```python
from build123d import *

# Parameters (mm, degrees)
SKETCH_1_R             = 1.5
EXTRUDE_1_DEPTH        = 8
SKETCH_2_R             = 1
CUT_EXTRUDE_1_DEPTH    = 33
FILLET_1_R             = 2
HOLE_WIZARD_M3_1_D     = 2.5
EXTRUDE_START          = 2.3
SKETCH_8_R             = 4.5
SKETCH_8_R_2           = 1.5
EXTRUDE_2_DEPTH        = 2.3
HOLE_WIZARD_M5_1_D     = 4.2
HOLE_WIZARD_M5_1_DEPTH = 20
HOLE_WIZARD_M5_1_TIP   = 1.2618073
CUT_EXTRUDE_2_DEPTH    = 20


with BuildPart() as part:
    # 草图1 → 凸台-拉伸1 (new body)
    with BuildSketch(Plane.XY):
        with BuildLine():
            Line((0.5, -13), (15.5, -13))
            Line((15.5, -13), (15.5, 13))
            Line((15.5, 13), (0.5, 13))
            Line((0.5, 13), (-4.159282148, 1.717664698))
            ThreePointArc((-4.159282148, 1.717664698), (-4.5, 0), (-4.159282148, -1.717664698))
            Line((-4.159282148, -1.717664698), (0.5, -13))
        make_face()
        Circle(SKETCH_1_R, mode=Mode.SUBTRACT)
    extrude(amount=EXTRUDE_1_DEPTH)

    # 草图2 → 切除-拉伸1 (cut)
    with BuildSketch(Plane.XY.offset(8)):
        with Locations((8.5, 10)):
            Circle(SKETCH_2_R)
        with Locations((8.5, -10)):
            Circle(SKETCH_2_R)
    extrude(amount=-CUT_EXTRUDE_1_DEPTH, mode=Mode.SUBTRACT)

    # 圆角1
    fillet_1_edges = [part.edges().sort_by_distance(p)[0] for p in [
        (0.5, 13, 4),
        (15.5, 13, 4),
        (15.5, -13, 4),
        (0.5, -13, 4),
    ]]
    fillet(fillet_1_edges, radius=FILLET_1_R)

    # M3 螺纹孔1 (through all)
    with Locations(Plane.XY.offset(8)):
        with Locations((8.5, 10), (8.5, -10)):
            Hole(HOLE_WIZARD_M3_1_D / 2)

    # 草图8 → 凸台-拉伸2 (add)
    with BuildSketch(Plane(origin=(0, 0, 0), x_dir=(-1, 0, 0), z_dir=(0, 0, -1)).offset(EXTRUDE_START)):
        Circle(SKETCH_8_R)
        Circle(SKETCH_8_R_2, mode=Mode.SUBTRACT)
    extrude(amount=-EXTRUDE_2_DEPTH)

    # M5 螺纹孔1
    with Locations(Plane.XY.offset(8)):
        with Locations((0, 0)):
            Hole(HOLE_WIZARD_M5_1_D / 2, depth=HOLE_WIZARD_M5_1_DEPTH)
            with Locations((0, 0, -(HOLE_WIZARD_M5_1_DEPTH + HOLE_WIZARD_M5_1_TIP / 2))):  # 118° drill point
                Cone(0, HOLE_WIZARD_M5_1_D / 2, HOLE_WIZARD_M5_1_TIP, mode=Mode.SUBTRACT)

    # 草图12 → 切除-拉伸2 (cut)
    with BuildSketch(Plane(origin=(0, 0, 0), x_dir=(-1, 0, 0), z_dir=(0, 0, -1))):
        with BuildLine():
            Line((-6, 4), (-6, -4))
            ThreePointArc((-6, -4), (-8.5, -6.5), (-11, -4))
            Line((-11, -4), (-11, 4))
            ThreePointArc((-11, 4), (-8.5, 6.5), (-6, 4))
        make_face()
    extrude(amount=-CUT_EXTRUDE_2_DEPTH, mode=Mode.SUBTRACT)


solid = part.part
```
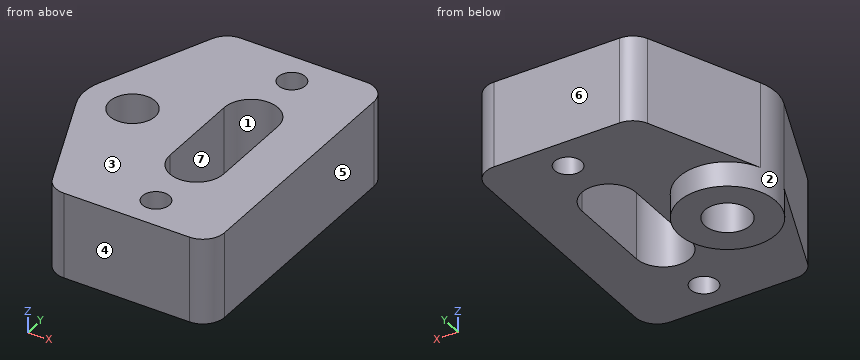
Input: part model. Units: mm. Frame: model coordinates. Face numbers are marked on the shaded views. A direction names the side the tool comes from. Round coordinates to 2 decimals unless told otherwise and drop trailing zeros. Loops run counter-clockwise (first coordinate to the right, second up) from the corner with the lowest first, then second, coordinate; pieces in that order, holes last. Notation, with made-up numbers: (21.25, 29) - (66.25, 29) arc R14 ccw to (66.25, 34) - close; hole circle Ø5 at (39, -37). An arc over 180 degrees is marked (long way). One line per item, written item: value. Start each with the question number.
(1) Section D-D, the plane z = -1. Return loops of the section in (x, y).
(2) Section B-B, the plane z = 2.25. Return loops of the section in (x, y).
(3) Draft query along Y for the marked faces 4, 5, 6 and 7. Return one class per face: +Y half, -Y half, draft (parallel to the pull), parting line (faces both ways), or undercut.
(4) Contact query for a flat-ended pin moving along its axis: P1, Ø1.5, axis at x = 6, y = -4, coming from the -Z side. Output: stop coordinate, or through.
(5) Section A-A, the plane y = 0. Return loops of the section in (x, z).
(6) Section C-C, the plane y = -10.5. Return loops of the section in (x, z), plus the area to 3 significant figures.
(7) Access query for the marked faces 1, 2 and 3. Directions: +Z, -Z, +X, -X, +Y, -Y. A direction counts if a zero-diameter tool reaches every point of the face in a straight line with its end or side. Return the directions, or none.
(8) Ray query, line 1 (Y direction, x = 8.5, z = 4.75); line 2 (X direction, y = 0.5, z = 1); line 3 (Y direction, x = 0, z = -1). Return the intervals inside material, ascending. Write a range as [from, to].
Results below:
1. outline: circle Ø9 at (0, 0); hole circle Ø4.2 at (0, 0)
2. outline: (-4.16, -1.72) - (-0.01, -11.76) arc R2 ccw to (1.84, -13) - (13.5, -13) arc R2 ccw to (15.5, -11) - (15.5, 11) arc R2 ccw to (13.5, 13) - (1.84, 13) arc R2 ccw to (-0.01, 11.76) - (-4.16, 1.72) arc R4.5 ccw to start; hole circle Ø4.2 at (0, 0); hole (6, -4) arc R2.5 ccw to (11, -4) - (11, 4) arc R2.5 ccw to (6, 4) - close; hole circle Ø2.5 at (8.5, -10); hole circle Ø2.5 at (8.5, 10)
3. face 4: -Y half
3. face 5: draft
3. face 6: +Y half
3. face 7: undercut
4. P1: z = 0
5. outline: (-4.5, -2.3) - (-2.1, -2.3) - (-2.1, 8) - (-4.5, 8) - close; (2.1, -2.3) - (4.5, -2.3) - (4.5, 0) - (6, 0) - (6, 8) - (2.1, 8) - close; (11, 0) - (15.5, 0) - (15.5, 8) - (11, 8) - close
6. outline: (-0.53, 0) - (7.35, 0) - (7.35, 8) - (-0.53, 8) - close; (9.65, 0) - (15.5, 0) - (15.5, 8) - (9.65, 8) - close
6. area: 110 mm^2
7. face 1: +Z, -Z
7. face 2: -Z
7. face 3: +Z, +X, -X, +Y, -Y
8. line 1: [-13, -11.25], [-8.75, -6.5], [6.5, 8.75], [11.25, 13]
8. line 2: [-4.47, -2.04], [2.04, 6], [11, 15.5]
8. line 3: [-4.5, -2.1], [2.1, 4.5]
